Here's how the part is built. I have some questions about the finished solid (model axes, mm). A direction names the side the tool comes from. Give positions to 0.01 mm unless a question says otherwise; leave off trailing zeros. Loops run counter-clockwise (first coordinate to the right, second up) from the corner with the lowest first, then second, coordinate; pieces in that order, holes last. Notation, with made-up numbers: (-27, 65.5) -> (-7, 65.5) arc R31 cw to (-7, 101.5) -> close; hole circle Ø9 at (-23.75, -34.5). An arc over 180 degrees is marked (long way). Answer in a Markdown table with one row per item. Add a question column.
Item 1: If we section it at D-D (y = -1.5): Write out the boundary of the cut face in (x, z), then the cut area to 3 significant figures.
Item 2: If we section it at C-C (z = 24): Write out the boundary of the cut face in (x, y).
Item 3: If we section it at B-B (x = -43): Write out the boundary of the cut face in (y, z), then the cut area to 3 significant figures.
Item 4: For P1, Ø2.5, axis at y = -5.4, z = 13.56, coming from the +X side; P2, Ø2, axis at y = 0, z = 19.5, coming from the -X side; P3, Ø1, axis at x = 14.5, z = 6, coming from the -Y side; P4, Ø4.5, axis at x = 6, z = 11, coming from the -Y side, each with a flat end and sliding along its axis, tell me the tip position at first contact or that it passes through.
Item 5: We'd pull the mould along Y, two halves only. Please class faces 6 (the face through (34, -3, 14)), 7 (the face through (-8, -3, 10)), 8 (the face through (-8, -3, 17)), 9 (the face through (-8, -1, 7.5)): released by +Y, released by -Y, zero draft, split by the parting line, or undercut.
Item 6: If I drill on line 1 (Y direction, x = 26, z = 8.25); line 2 (Z direction, x = -18, y = -5.25); line 3 (Y direction, x = -38, z = 6.5), over which ranges is the centre line in solid material (lowest first)?
Item 7: Which directions (+Z, -Z, +X, -X, +Y, -Y) give clear straight access to the entire face, cutting with the end or side of a thin tool? Please do faces 1 (the face through (32.33, -1, 13)), 2 (the face through (-50, -4, 12)), 3 (the face through (-8, -1, 19.5)), 4 (the face through (-8, 0, 4)), 5 (the face through (35, -4, 15)).
Item 8: If we section it at A-A (y = -6): Write out the boundary of the cut face in (x, z).
```python
from build123d import *

# Parameters (mm, degrees)
F0_W      = 80
F0_H      = 6
F1_DEPTH  = 3
F0_H_2    = 7.5
F2_DEPTH  = 1
F3_R      = 2.5
F3_R_2    = 1.5
F4_DEPTH  = 50
F4_FACE_R = 1.5
F5_DEPTH  = 35


with BuildPart() as f1:
    # F0 (on Front) → F1 (new body)
    with BuildSketch(Plane.XZ):
        with Locations((-7.669735, 16.5)):
            Rectangle(F0_W, F0_H)
        with Locations((-7.669735, 10.5)):
            Rectangle(F0_W, F0_H)
    extrude(amount=F1_DEPTH)

    # F0 (on Front) → F2 (join)
    with BuildSketch(Plane.XZ):
        with Locations((-7.669735, 23.25)):
            Rectangle(F0_W, F0_H_2)
        with Locations((-7.669735, 3.75)):
            Rectangle(F0_W, F0_H_2)
        with Locations((-7.669735, 10.5)):
            Rectangle(F0_W, F0_H)
        with Locations((-7.669735, 16.5)):
            Rectangle(F0_W, F0_H)
    extrude(amount=-F2_DEPTH)

    # F3 (on Right) → F4 (join)
    with BuildSketch(Plane.YZ):
        with Locations((-5.398772, 13.555951)):
            Circle(F3_R)
        with Locations((-5.398772, 13.555951)):
            Circle(F3_R_2, mode=Mode.SUBTRACT)
    extrude(amount=-F4_DEPTH)

    # F4_face (on face) → F5 (join)
    with BuildSketch(Plane(origin=(0, -5.41744, 13.555951), x_dir=(0, 1, 0), z_dir=(1, 0, 0))):
        with BuildLine():
            Line((2.41744, -0.704196), (2.41744, 0.704196))
            ThreePointArc((2.41744, 0.704196), (-2.481332, 0), (2.41744, -0.704196))
        make_face()
        with Locations((0.018668, 0)):
            Circle(F4_FACE_R, mode=Mode.SUBTRACT)
    extrude(amount=F5_DEPTH)


solid = f1.part
```
Recorded:
| question | item | result |
|---|---|---|
| 1 | outline | (-47.67, 7.5) -> (32.33, 7.5) -> (32.33, 19.5) -> (-47.67, 19.5) -> close |
| 1 | area | 960 mm^2 |
| 2 | outline | (-47.67, 0) -> (32.33, 0) -> (32.33, 1) -> (-47.67, 1) -> close |
| 3 | outline | (-3, 7.5) -> (0, 7.5) -> (0, 0) -> (1, 0) -> (1, 27) -> (0, 27) -> (0, 19.5) -> (-3, 19.5) -> (-3, 14.26) arc R2.5 ccw (long way) to (-3, 12.85) -> close; hole circle Ø3 at (-5.4, 13.56) |
| 3 | area | 75.5 mm^2 |
| 4 | P1 | passes through |
| 4 | P2 | stops at x = -47.67 |
| 4 | P3 | stops at y = 0 |
| 4 | P4 | stops at y = -7.88 |
| 5 | face 6 | released by +Y |
| 5 | face 7 | undercut |
| 5 | face 8 | undercut |
| 5 | face 9 | zero draft |
| 6 | line 1 | y = -3 to 1 |
| 6 | line 2 | z = 11.06 to 12.06, 15.05 to 16.05 |
| 6 | line 3 | y = 0 to 1 |
| 7 | face 1 | +Z, -Z, +X, +Y |
| 7 | face 2 | +Z, -Z, -X, +Y, -Y |
| 7 | face 3 | +Z, +X, -X, -Y |
| 7 | face 4 | -Z, +X, -X, -Y |
| 7 | face 5 | +Z, -Z, +X, +Y, -Y |
| 8 | outline | (-50, 11.13) -> (35, 11.13) -> (35, 12.18) -> (-50, 12.18) -> close; (-50, 14.93) -> (35, 14.93) -> (35, 15.98) -> (-50, 15.98) -> close |
